Build history of the part. All positions in model axes, mm. A direction names the side the tool comes from. Coordinates: 2 decimals unless noted, no trailing zeros. Order: outer loops, then holes, each group sorted by start corner. A loop starts at its lowest first (then second) coordinate and runs counter-clockwise, first axis right, second up. Notation, with made-up numbers: (-9.5, 82.25) - (21.5, 82.25) arc R11 ccw to (21.5, 98.25) - close; hole circle Ø8 at (-25, -28). An arc over 180 degrees is marked (long way). One line per item, written item: value.
from build123d import *

# Parameters (mm, degrees)
ESQUISSE6_R                                   = 18.8595
BOSS_EXTRU_2_DEPTH                            = 25.4
ESQUISSE7_R                                   = 17.78
BOSS_EXTRU_3_DEPTH                            = 30.48
ESQUISSE8_R                                   = 17.145
BOSS_EXTRU_4_DEPTH                            = 15.4432
ESQUISSE9_R                                   = 5.969
BOSS_EXTRU_5_DEPTH                            = 6.096
ESQUISSE10_R                                  = 4.699
BOSS_EXTRU_6_DEPTH                            = 4.233333333
ESQUISSE11_R                                  = 11.0617
BOSS_EXTRU_7_DEPTH                            = 6.35
ESQUISSE12_R                                  = 4.7752
BOSS_EXTRU_8_DEPTH                            = 3.302
PER_AGE_POUR_TUYAU_POUR_TROU_TARAUD_1_1_D     = 6.1468
PER_AGE_POUR_TUYAU_POUR_TROU_TARAUD_1_1_DEPTH = 19.981333333
BOSS_EXTRU_9_DEPTH                            = 19.981333333
BOSS_EXTRU_10_DEPTH                           = 2.032
ENL_V_MAT_EXTRU_2_REACH                       = 93.955
ESQUISSE18_R                                  = 1.4605
ESQUISSE19_R                                  = 1.5
ESQUISSE19_R_2                                = 1.500000048
ENL_V_MAT_EXTRU_3_DEPTH                       = 5


with BuildPart() as part:
    # Esquisse6 → Boss.-Extru.2 (new body)
    with BuildSketch(Plane(origin=(0, 0, 0), x_dir=(0, 0, -1), z_dir=(1, 0, 0))):
        Circle(ESQUISSE6_R)
    extrude(amount=BOSS_EXTRU_2_DEPTH)

    # Esquisse7 → Boss.-Extru.3 (add)
    with BuildSketch(Plane(origin=(25.4, 0, 0), x_dir=(0, 0, -1), z_dir=(1, 0, 0))):
        with Locations(Location((0, 0, 0), (0, 0, 180))):
            Circle(ESQUISSE7_R)
    extrude(amount=BOSS_EXTRU_3_DEPTH)

    # Esquisse8 → Boss.-Extru.4 (add)
    with BuildSketch(Plane(origin=(55.88, 0, 0), x_dir=(0, 0, -1), z_dir=(1, 0, 0))):
        with Locations(Location((0, 0, 0), (0, 0, 180))):
            Circle(ESQUISSE8_R)
    extrude(amount=BOSS_EXTRU_4_DEPTH)

    # Esquisse9 → Boss.-Extru.5 (add)
    with BuildSketch(Plane.ZY):
        with Locations(Location((0, -6.35, 0), (0, 0, 180))):
            Circle(ESQUISSE9_R)
    extrude(amount=BOSS_EXTRU_5_DEPTH)

    # Esquisse10 → Boss.-Extru.6 (add)
    with BuildSketch(Plane.ZY.offset(6.096)):
        with Locations((0, -6.35)):
            Circle(ESQUISSE10_R)
    extrude(amount=BOSS_EXTRU_6_DEPTH)

    # Esquisse11 → Boss.-Extru.7 (add)
    with BuildSketch(Plane.ZY.offset(10.329333333)):
        with Locations((0, -6.35)):
            Circle(ESQUISSE11_R)
    extrude(amount=BOSS_EXTRU_7_DEPTH)

    # Esquisse12 → Boss.-Extru.8 (add)
    with BuildSketch(Plane.ZY.offset(16.679333333)):
        with Locations(Location((0, -6.35, 0), (0, 0, 180))):
            Circle(ESQUISSE12_R)
    extrude(amount=BOSS_EXTRU_8_DEPTH)

    # Perçage pour tuyau pour trou taraudé 1/161
    with Locations(Plane.ZY.offset(19.981333333)):
        with Locations((0, -6.35)):
            Hole(PER_AGE_POUR_TUYAU_POUR_TROU_TARAUD_1_1_D / 2, depth=PER_AGE_POUR_TUYAU_POUR_TROU_TARAUD_1_1_DEPTH)

    # Esquisse16 → Boss.-Extru.9 (add)
    with BuildSketch(Plane.ZY):
        with BuildLine():
            Line((-1.778, -3.968758467), (1.778, -3.968758467))
            ThreePointArc((1.778, -3.968758467), (0, -9.3218), (-1.778, -3.968758467))
        make_face()
    extrude(amount=BOSS_EXTRU_9_DEPTH)

    # Esquisse17 → Boss.-Extru.10 (add)
    with BuildSketch(Plane.ZY.offset(19.981333333)):
        with BuildLine():
            Line((-1.778, -3.968758467), (1.778, -3.968758467))
            ThreePointArc((1.778, -3.968758467), (0, -9.3218), (-1.778, -3.968758467))
        make_face()
    extrude(amount=BOSS_EXTRU_10_DEPTH)

    # Esquisse18 → Enlèv. mat.-Extru.2 (cut, up to next)
    with BuildSketch(Plane.ZY.offset(16.679333333), mode=Mode.PRIVATE) as enl_v_mat_extru_2_sk1:
        with Locations((0, 0.254)):
            Circle(ESQUISSE18_R)
    enl_v_mat_extru_2_tool1 = extrude(enl_v_mat_extru_2_sk1.sketch, amount=-ENL_V_MAT_EXTRU_2_REACH, mode=Mode.PRIVATE) & part.part
    # Esquisse18 → Enlèv. mat.-Extru.2 (cut, up to next)
    with BuildSketch(Plane.ZY.offset(16.679333333), mode=Mode.PRIVATE) as enl_v_mat_extru_2_sk2:
        with Locations((6.604, -6.35)):
            Circle(ESQUISSE18_R)
    enl_v_mat_extru_2_tool2 = extrude(enl_v_mat_extru_2_sk2.sketch, amount=-ENL_V_MAT_EXTRU_2_REACH, mode=Mode.PRIVATE) & part.part
    # Esquisse18 → Enlèv. mat.-Extru.2 (cut, up to next)
    with BuildSketch(Plane.ZY.offset(16.679333333), mode=Mode.PRIVATE) as enl_v_mat_extru_2_sk3:
        with Locations((0, -12.954)):
            Circle(ESQUISSE18_R)
    enl_v_mat_extru_2_tool3 = extrude(enl_v_mat_extru_2_sk3.sketch, amount=-ENL_V_MAT_EXTRU_2_REACH, mode=Mode.PRIVATE) & part.part
    # Esquisse18 → Enlèv. mat.-Extru.2 (cut, up to next)
    with BuildSketch(Plane.ZY.offset(16.679333333), mode=Mode.PRIVATE) as enl_v_mat_extru_2_sk4:
        with Locations((-6.604, -6.35)):
            Circle(ESQUISSE18_R)
    enl_v_mat_extru_2_tool4 = extrude(enl_v_mat_extru_2_sk4.sketch, amount=-ENL_V_MAT_EXTRU_2_REACH, mode=Mode.PRIVATE) & part.part
    add(enl_v_mat_extru_2_tool1.solids().sort_by_distance((-16.679333, 0.254, 0))[0], mode=Mode.SUBTRACT)
    add(enl_v_mat_extru_2_tool2.solids().sort_by_distance((-16.679333, -6.35, 6.604))[0], mode=Mode.SUBTRACT)
    add(enl_v_mat_extru_2_tool3.solids().sort_by_distance((-16.679333, -12.954, 0))[0], mode=Mode.SUBTRACT)
    add(enl_v_mat_extru_2_tool4.solids().sort_by_distance((-16.679333, -6.35, -6.604))[0], mode=Mode.SUBTRACT)

    # Esquisse19 → Enlèv. mat.-Extru.3 (cut)
    with BuildSketch(Plane.ZY):
        with Locations((6.376248943, 14.789374018)):
            Circle(ESQUISSE19_R)
        with Locations((7.253318149, -15.510625982)):
            Circle(ESQUISSE19_R_2)
        with Locations((-16.809397398, 1.555003695)):
            Circle(ESQUISSE19_R_2)
    extrude(amount=-ENL_V_MAT_EXTRU_3_DEPTH, mode=Mode.SUBTRACT)


solid = part.part
1. Band-saw the part on B-B, the plane x = 7. Give the cut face in (y, z).
Values found:
outline: circle Ø37.72 at (0, 0)
2. Band-saw the part on A-A, the plane z = -14. Give the cut face in (x, y).
Values found:
outline: (0, -12.64) - (25.4, -12.64) - (25.4, -10.96) - (55.88, -10.96) - (55.88, -9.9) - (71.32, -9.9) - (71.32, 9.9) - (55.88, 9.9) - (55.88, 10.96) - (25.4, 10.96) - (25.4, 12.64) - (0, 12.64) - close
3. 3-axis set-ups, long thin cutter, end or side, ignore diameter. For faces 1 (the face through (40.43, 17.36, -3.85)), 2 (the face through (-16.679, -9, 5)), 3 (the face through (-8.183, -10.937, -1.019)): which of +Z, -Z, +X, -X, +Y, -Y reach the whole face in a straight line?
Values found:
face 1: +X
face 2: -X
face 3: none
4. Probe line 1 along X through (y, z) = (-14.5, -6.5); line 2 along X through (y, z) = (-2.5, 4.5); line 3 along X through (y, z) = (-2.5, 13). List the from-to ranges inside material, lowest first.
Values found:
line 1: x = -16.68 to -10.33, 0 to 71.32
line 2: x = -16.68 to -10.33, -6.1 to 71.32
line 3: x = 0 to 71.32
5. Two-plate mould, pull along Y, no slides. Class faces 4 (the face through (55.88, -15, -9)), 5 (the face through (-3.005, -12.268, 0.777)), 6 (the face through (2.465, 1.621, -18.308)), 7 (the face through (-13.55, 1.24, -1.08)): pulls with the +Y half, pulls with the -Y half, needs draft (parallel to the pull), parting line crosses it, or undercut.
Values found:
face 4: needs draft
face 5: parting line crosses it
face 6: undercut
face 7: undercut
6. Flat gauge pins, fed straight in: P1, Ø3, axis at x = 57.5, z = 12.5, coming from the -Y side; P2, Ø3, axis at x = 29.5, z = -14, coming from the -Y side; P3, Ø2.5, axis at y = 0.254, z = 0, coming from the -X side. Where does each tip first touch, or does it go through?
Values found:
P1: stops at y = -13.15
P2: stops at y = -12.64
P3: stops at x = -6.1
7. Band-saw the part on C-C, the plane y = -6.35. Count the separate pieces of the cut face and the enclosed holes in it, and give its area (3 significant figures).
Values found:
separate pieces: 3
enclosed holes: 0
area: 2,660 mm2
